```python
from build123d import *

# Parameters (mm, degrees)
BODYSKE_R  = 0.6
BODY_DEPTH = 0.9


with BuildPart() as part:
    # BodySke → Body (new body)
    with BuildSketch(Plane.XY):
        with BuildLine():
            Line((0.166935484, -8.048268916), (0.225, -10.8476668))
            Line((0.225, -10.8476668), (2.353032971, -10.803527592))
            ThreePointArc((2.353032971, -10.803527592), (2.676217488, -10.676116355), (2.838386738, -10.368898209))
            Line((2.838386738, -10.368898209), (2.936405186, -9.624374178))
            ThreePointArc((2.936405186, -9.624374178), (3.251364406, -8.851047556), (3.904664808, -8.331016828))
            ThreePointArc((3.904664808, -8.331016828), (0, 10.15), (-3.904664808, -8.331016828))
            ThreePointArc((-3.904664808, -8.331016828), (-3.251364406, -8.851047556), (-2.936405186, -9.624374178))
            Line((-2.936405186, -9.624374178), (-2.838386738, -10.368898209))
            ThreePointArc((-2.838386738, -10.368898209), (-2.676217488, -10.676116355), (-2.353032971, -10.803527592))
            Line((-2.353032971, -10.803527592), (-0.225, -10.8476668))
            Line((-0.225, -10.8476668), (-0.166935484, -8.048268916))
            ThreePointArc((-0.166935484, -8.048268916), (0, 8.05), (0.166935484, -8.048268916))
        make_face()
        with Locations((1.05, -9.61785449)):
            Circle(BODYSKE_R, mode=Mode.SUBTRACT)
        with Locations((-1.05, -9.61785449)):
            Circle(BODYSKE_R, mode=Mode.SUBTRACT)
    extrude(amount=-BODY_DEPTH)


solid = part.part
```
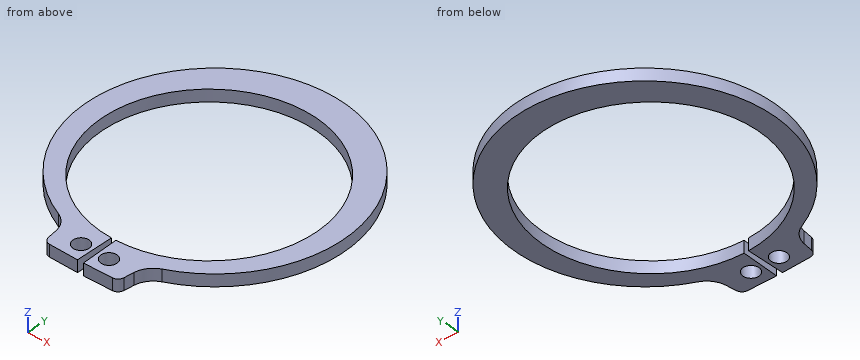
CAD build for the part. Positions are in the model's coordinates, mm. Coordinates: 2 decimals unless noted, no trailing zeros. Order: outer loops, then holes, each group sorted by start corner. A loop starts at its lowest first (then second) coordinate and runs counter-clockwise, first axis right, second up. Notation, with made-up numbers: M 35.5,-30.5 L 76.5,-30.5 A9 ccw 76.5,-23.5 Z; hole C 88.25,59 d2. An arc over 180 degrees is marked long. Write each question's results on one line, items separated by ' | '. Start each with the question number.
Q1. Drill centre lines: probe 1 along X at (y, z) = (0.25, -0.75); probe 2 along Y at (x, z) = (1.05, -0.6); probe 3 along X at (y, z) = (3.75, -0.65). Where is each one in solid material? Low to high. Write a range as from..to.
Q2. Flat gauge pin, fed straight in: P1, Ø1, axis at x = 2.5, y = -6, coming from the -Z side. Where does the tip first touch, or does it go through?
Q3. Cut at A-A (y = 2). List the corners of the cut face in (x, z).
Q4. Cut at C-C (z = -0.5). List the corners of the cut face in (x, y) (3 decimals), then the cut area to 3 significant figures.
Q5. Cut at D-D (x = 1.05). List the corners of the cut face in (y, z).
Q6. Cut at B-B (x = 5.25). List the corners of the cut face in (y, z), then the cut area to 3 significant figures.
Found:
1) probe 1: -9.65..-8.05, 8.05..9.65 | probe 2: -10.83..-10.22, -9.02..-7.98, 7.98..10.09 | probe 3: -9.09..-7.12, 7.12..9.09
2) P1: through
3) outline: M -9.54,-0.9 L -7.8,-0.9 L -7.8,0 L -9.54,0 Z; M 7.8,-0.9 L 9.54,-0.9 L 9.54,0 L 7.8,0 Z
4) outline: M -3.905,-8.331 A1.65 cw -2.936,-9.624 L -2.838,-10.369 A0.5 ccw -2.353,-10.804 L -0.225,-10.848 L -0.167,-8.048 A8.05 cw long 0.167,-8.048 L 0.225,-10.848 L 2.353,-10.804 A0.5 ccw 2.838,-10.369 L 2.936,-9.624 A1.65 cw 3.905,-8.331 A9.653 ccw long Z; hole C -1.05,-9.618 d1.2; hole C 1.05,-9.618 d1.2 | area: 96.6 mm²
5) outline: M -10.83,-0.9 L -10.22,-0.9 L -10.22,0 L -10.83,0 Z; M -9.02,-0.9 L -7.98,-0.9 L -7.98,0 L -9.02,0 Z; M 7.98,-0.9 L 10.09,-0.9 L 10.09,0 L 7.98,0 Z
6) outline: M -7.6,-0.9 L -6.1,-0.9 L -6.1,0 L -7.6,0 Z; M 6.1,-0.9 L 8.6,-0.9 L 8.6,0 L 6.1,0 Z | area: 3.60 mm²
